Could you check a few things on this model? Use its own coordinates, in mm. A direction names the side the tool comes from. Round coordinates to 2 decimals unless told otherwise and drop trailing zeros. Write each loop counter-clockwise with the first axis right and the second up, starting at its lowest first coordinate (ties: lowest second). Pieces come first, ordered by that corner, then holes. Notation, with made-up numbers: M 50,37.25 L 97,37.25 A7 ccw 97,46.25 Z; hole C -7.75,41.5 d5. An arc over 180 degrees is marked long. One line per item, written item: value. Start each with the question number.
(1) If I drill on L1, parallel to X at y = -2.5, z = -7; L2, parallel to Y at x = -2, z = -1; L3, parallel to Z at x = -0.25, y = 3.5, over which ranges is the centre line in solid material (lowest first)?
(2) I want a section at D-D on y = -3.25. Please give me the cut outline in (x, z), and give its area (3 significant figures).
(3) Which directions (+Z, -Z, +X, -X, +Y, -Y) give clear straight access to the entire face, cutting with the end or side of a thin tool? Please do faces 4 (the face through (-3, -3, -1.4)), 5 (the face through (-3, 0, -2.9)), 6 (the face through (2.9, 0, -7)), 7 (the face through (2.2, -3, -7)), 8 (the face through (1, -3, -2.6)).
(4) I'm going to push a flat-ended pin straight in: pin 1 Ø0.9 at (x, y) = (-3, -3) entering from +Z. Where does the tip first touch, or does it pass through?
(5) I want a section at A-A on y = 0. Please give me the cut outline in (x, z), and give its area (3 significant figures).
(6) I want a section at B-B on z = -6.25. Please give me the cut outline in (x, y).
(7) I want a section at C-C on x = -2.75. Please give me the cut outline in (y, z).
(8) Thinking about a two-plate mould opening in Y: for faces 1 (the face through (1.2, -3, -6)), 2 (the face through (0, 3.9, -4)), 3 (the face through (-0.041, -0.029, -3.682)), which applies, released by +Y, released by -Y, zero draft, split by the parting line, or undercut?
```python
from build123d import *

# Parameters (mm, degrees)
SKETCH001_W     = 7.8
SKETCH001_H     = 7.8
PAD_DEPTH       = 7.5
POCKET_DEPTH    = 2.1
POCKET001_DEPTH = 5


with BuildPart() as part:
    # Sketch → Revolution (revolve)
    with BuildSketch(Plane.XZ):
        with BuildLine():
            Line((0, 0), (0, 2))
            Line((0, 2), (-2.1, 2))
            ThreePointArc((-2.1, 2), (-2.382843, 1.882843), (-2.5, 1.6))
            Line((-2.5, 1.6), (-2.5, 0))
            Line((-2.5, 0), (0, 0))
        make_face()
    revolve(axis=Axis((0, 0, 0), (0, 0, 1)))

    # Sketch001 → Pad (new body)
    with BuildSketch(Plane.XY):
        Rectangle(SKETCH001_W, SKETCH001_H)
    extrude(amount=-PAD_DEPTH)

    # Sketch002 → Pocket (cut, symmetric)
    with BuildSketch(Plane.XZ):
        with BuildLine():
            Line((-3.9, -0.7), (-1.9, -0.7))
            ThreePointArc((2.9, -5.5), (1.494113, -2.105887), (-1.9, -0.7))
            Line((2.9, -7.5), (2.9, -5.5))
            Line((0.7, -7.5), (2.9, -7.5))
            Line((0.7, -7.5), (0.7, -5.5))
            ThreePointArc((0.7, -5.5), (-0.061522, -3.661522), (-1.9, -2.9))
            Line((-3.9, -2.9), (-1.9, -2.9))
            Line((-3.9, -0.7), (-3.9, -2.9))
        make_face()
    extrude(amount=POCKET_DEPTH, both=True, mode=Mode.SUBTRACT)

    # Sketch003 → Pocket001 (cut)
    with BuildSketch(Plane.XZ):
        with BuildLine():
            Line((-1.9, -1.4), (-3.9, -1.4))
            Line((-3.9, -1.4), (-3.9, -2.4))
            Line((-3.9, -2.4), (-1.9, -2.4))
            ThreePointArc((1.2, -5.5), (0.292031, -3.307969), (-1.9, -2.4))
            Line((1.2, -5.5), (1.2, -7.5))
            Line((1.2, -7.5), (2.2, -7.5))
            Line((2.2, -7.5), (2.2, -5.5))
            ThreePointArc((2.2, -5.5), (0.999138, -2.600862), (-1.9, -1.4))
        make_face()
    extrude(amount=POCKET001_DEPTH, mode=Mode.SUBTRACT)


solid = part.part
```
Found:
1. L1: x = -3.9 to 1.2, 2.2 to 3.9
1. L2: y = -3.9 to -2.1, 2.1 to 3.9
1. L3: z = -7.5 to 0
2. outline: M -3.9,-7.5 L 1.2,-7.5 L 1.2,-5.5 A3.1 ccw -1.9,-2.4 L -3.9,-2.4 Z; M -3.9,-1.4 L -1.9,-1.4 A4.1 cw 2.2,-5.5 L 2.2,-7.5 L 3.9,-7.5 L 3.9,0 L -3.9,0 Z
2. area: 48.8 mm²
3. face 4: -X, -Y
3. face 5: -X
3. face 6: -Z
3. face 7: -Z, -Y
3. face 8: -Y
4. pin 1: stops at z = 0
5. outline: M -3.9,-7.5 L 0.7,-7.5 L 0.7,-5.5 A2.6 ccw -1.9,-2.9 L -3.9,-2.9 Z; M -3.9,-0.7 L -1.9,-0.7 A4.8 cw 2.9,-5.5 L 2.9,-7.5 L 3.9,-7.5 L 3.9,0 L 2.5,0 L 2.5,1.6 A0.4 ccw 2.1,2 L -2.1,2 A0.4 ccw -2.5,1.6 L -2.5,0 L -3.9,0 Z
5. area: 46.8 mm²
6. outline: M -3.9,-3.9 L 1.2,-3.9 L 1.2,-2.1 L 0.7,-2.1 L 0.7,2.1 L 2.9,2.1 L 2.9,-2.1 L 2.2,-2.1 L 2.2,-3.9 L 3.9,-3.9 L 3.9,3.9 L -3.9,3.9 Z
7. outline: M -3.9,-7.5 L 3.9,-7.5 L 3.9,0 L -3.9,0 L -3.9,-1.4 L -2.1,-1.4 L -2.1,-0.7 L 2.1,-0.7 L 2.1,-2.9 L -2.1,-2.9 L -2.1,-2.4 L -3.9,-2.4 Z
8. face 1: zero draft
8. face 2: released by +Y
8. face 3: undercut
